from build123d import *

# Parameters (mm, degrees)
F0_R     = 12.5
F0_R_2   = 4
F1_DEPTH = 2
F2_R     = 9.5
F2_R_2   = 4
F3_DEPTH = 2
F4_SIZE  = 0.25


with BuildPart() as f1:
    # F0 (on Top) → F1 (new body)
    with BuildSketch(Plane.XY):
        Circle(F0_R)
        Circle(F0_R_2, mode=Mode.SUBTRACT)
    extrude(amount=F1_DEPTH)

    # F2 (on face) → F3 (join)
    with BuildSketch(Plane.XY.offset(2)):
        Circle(F2_R)
        Circle(F2_R_2, mode=Mode.SUBTRACT)
    extrude(amount=F3_DEPTH)

    # F4
    f4_edges = [f1.edges().sort_by_distance(p)[0] for p in [
        (-9.5, 0, 4),
        (-4, 0, 4),
        (-12.5, 0, 2),
        (-12.5, 0, 0),
        (-4, 0, 0),
    ]]
    chamfer(f4_edges, length=F4_SIZE)


solid = f1.part
Could you check a few things on this model? Use its own coordinates, in mm. A direction names the side the tool comes from. Round coordinates to 2 decimals unless told otherwise and drop trailing zeros. Write each loop counter-clockwise with the first axis right and the second up, starting at its lowest first coordinate (ties: lowest second). Pieces come first, ordered by that corner, then holes. Notation, with made-up numbers: (24, -32.75) - (75, -32.75) arc R12 ccw to (75, -24.75) - close; hole circle Ø2 at (33.25, 20.25). An arc over 180 degrees is marked (long way). Put each result on its own line as item: value. Start each with the question number.
(1) I want a section at C-C, the plane z = 2.65. Please give me the cut outline in (x, y), plus the area to 3 significant figures.
(2) Will this pin go through, and if not, where does the flat tip stop? pin 1 (2 mm diameter, centred on x = 3, z = 2, fed in from -Y).
(3) For faces 4 (the flat face through (5, 0, 0)), 5 (the flat face through (4, -9, 2)), which set-ups out of +Z, -Z, +X, -X, +Y, -Y let a thin tool reach every point of the face, with its end or its side?
(4) Thinking about a two-plate mould opening in Y: for faces 1 (the flat face through (4, -2, 4)), 2 (the cylindrical face through (4.38, -8.43, 2.86)), 3 (the cylindrical face through (-0.867, -3.905, 1.976)), which applies, released by +Y, released by -Y, zero draft, split by the parting line, or undercut?
(5) I want a section at A-A, the plane x = 0. Please give me the cut outline in (y, z), plus the area to 3 significant figures.
(6) I need wall thicknesses on probe 1 along Y at (x, z) = (0, 2.9); probe 2 along Y at (x, z) = (0, 1.5); probe 3 along Z at (x, y) = (-10, -2.5). Which ranges of each line are inside material? Lowest first, please.
Here are the results:
1. outline: circle Ø19 at (0, 0); hole circle Ø8 at (0, 0)
1. area: 233 mm^2
2. pin 1: stops at y = -12.33
3. face 4: -Z, +X, -X, +Y, -Y
3. face 5: +Z
4. face 1: zero draft
4. face 2: split by the parting line
4. face 3: undercut
5. outline: (-12.5, 0.25) - (-12.25, 0) - (-4.25, 0) - (-4, 0.25) - (-4, 3.75) - (-4.25, 4) - (-9.25, 4) - (-9.5, 3.75) - (-9.5, 2) - (-12.25, 2) - (-12.5, 1.75) - close; (4, 0.25) - (4.25, 0) - (12.25, 0) - (12.5, 0.25) - (12.5, 1.75) - (12.25, 2) - (9.5, 2) - (9.5, 3.75) - (9.25, 4) - (4.25, 4) - (4, 3.75) - close
5. area: 55.7 mm^2
6. probe 1: y = -9.5 to -4, 4 to 9.5
6. probe 2: y = -12.5 to -4, 4 to 12.5
6. probe 3: z = 0 to 2
